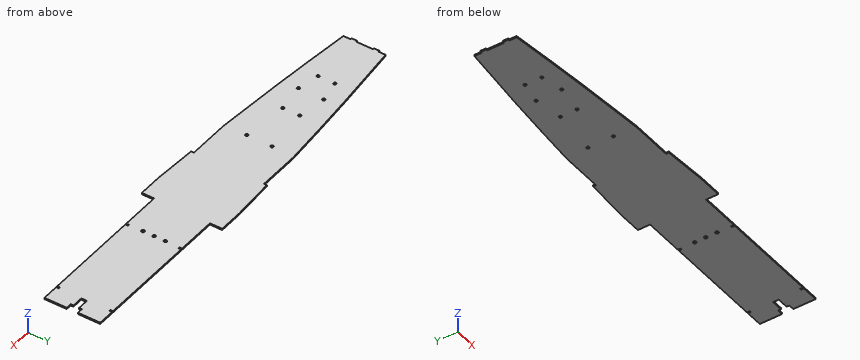
```python
from build123d import *

# Parameters (mm, degrees)
BOSS_EXTRUDE1_DEPTH    = 1.5875
CUT_EXTRUDE1_DEPTH     = 637.645771754
SKETCH4_W              = 1.5875
SKETCH4_H              = 3.175
CUT_EXTRUDE2_DEPTH     = 637.645771754
SKETCH6_W              = 47.338109293
SKETCH6_H              = 3.175
CUT_EXTRUDE3_DEPTH     = 637.645771754
SKETCH7_R              = 1.5875
ARTS4_MOUNT_DEPTH      = 637.645771754
SKETCH8_R              = 1.5875
TELEMETRUM_MOUNT_DEPTH = 637.645771754
SKETCH9_R              = 1.74625
CUT_EXTRUDE4_DEPTH     = 637.645771754


with BuildPart() as part:
    # Sketch1 → Boss-Extrude1 (new body)
    with BuildSketch(Plane.XY):
        with BuildLine():
            Line((508, -45.72), (508, -34.29))
            Line((508, -34.29), (635, -34.29))
            Line((635, -34.29), (635, 34.29))
            Line((635, 34.29), (508, 34.29))
            Line((508, 34.29), (508, 45.72))
            Line((508, 45.72), (429.947642932, 45.72))
            add(Edge.make_bspline(
                [(161.29, 23.981640211), (161.616784041, 24.018741883), (172.383373415, 25.239568053), (204.048179593, 28.679227521), (256.348102033, 33.727983978), (319.188209115, 38.915614913), (371.60802888, 42.52482202), (408.536828327, 44.644949518), (424.488578703, 45.455997775), (429.947642932, 45.72)],
                knots=[0.31962734, 0.31962734, 0.31962734, 0.31962734, 0.321557959, 0.383234508, 0.506587607, 0.629940705, 0.753293803, 0.814970352, 0.847054623, 0.847054623, 0.847054623, 0.847054623], degree=3))
            Line((161.29, 23.981640211), (161.29, 15.875))
            Line((161.29, 15.875), (159.7025, 15.875))
            Line((159.7025, 15.875), (159.7025, 9.525))
            Line((159.7025, 9.525), (161.29, 9.525))
            Line((161.29, 9.525), (161.29, -9.525))
            Line((161.29, -9.525), (159.7025, -9.525))
            Line((159.7025, -9.525), (159.7025, -15.875))
            Line((159.7025, -15.875), (161.29, -15.875))
            Line((161.29, -15.875), (161.29, -23.981640211))
            add(Edge.make_bspline(
                [(429.947642932, -45.72), (424.488578703, -45.455997775), (408.536828327, -44.644949518), (371.60802888, -42.52482202), (319.188209115, -38.915614913), (256.348102033, -33.727983978), (204.048179593, -28.679227521), (172.383373415, -25.239568053), (161.616784041, -24.018741883), (161.29, -23.981640211)],
                knots=[0.16612059, 0.16612059, 0.16612059, 0.16612059, 0.198204861, 0.25988141, 0.383234508, 0.506587607, 0.629940705, 0.691617254, 0.693547873, 0.693547873, 0.693547873, 0.693547873], degree=3))
            Line((429.947642932, -45.72), (508, -45.72))
        make_face()
    extrude(amount=BOSS_EXTRUDE1_DEPTH)

    # Sketch3 → Cut-Extrude1 (cut, through all)
    with BuildSketch(Plane.XY.offset(1.5875)):
        Polygon((635, 34.29), (508, 34.29), (508, 45.72), (457.2, 45.72), (457.2, 31.75), (635, 31.75), align=None)
        Polygon((508, -45.72), (508, -34.29), (635, -34.29), (635, -31.75), (457.2, -31.75), (457.2, -45.72), align=None)
        Polygon((628.65, 6.35), (628.65, 3.175), (615.95, 3.175), (615.95, -3.175), (628.65, -3.175), (628.65, -6.35), (635, -6.35), (635, 6.35), align=None)
    extrude(amount=-CUT_EXTRUDE1_DEPTH, mode=Mode.SUBTRACT)

    # Sketch4 → Cut-Extrude2 (cut, through all)
    with BuildSketch(Plane.XY.offset(1.5875)):
        with Locations((503.1105, 30.1625)):
            Rectangle(SKETCH4_W, SKETCH4_H)
        with Locations((615.15625, 30.1625)):
            Rectangle(SKETCH4_W, SKETCH4_H)
        with Locations((503.1105, -30.1625)):
            Rectangle(SKETCH4_W, SKETCH4_H)
        with Locations((615.15625, -30.1625)):
            Rectangle(SKETCH4_W, SKETCH4_H)
    extrude(amount=-CUT_EXTRUDE2_DEPTH, mode=Mode.SUBTRACT)

    # Sketch6 → Cut-Extrude3 (cut, through all)
    with BuildSketch(Plane.XY.offset(1.5875)):
        with Locations((357.330945353, 41.432202354)):
            Rectangle(SKETCH6_W, SKETCH6_H)
        with Locations((357.330945353, -41.432202354)):
            Rectangle(SKETCH6_W, SKETCH6_H)
    extrude(amount=-CUT_EXTRUDE3_DEPTH, mode=Mode.SUBTRACT)

    # Sketch7 → ARTS4 mount (cut, through all)
    with BuildSketch(Plane.XY.offset(1.5875)):
        with Locations((331.688780886, 14.478)):
            Circle(SKETCH7_R)
        with Locations((331.688780886, -14.478)):
            Circle(SKETCH7_R)
        with Locations((247.868780886, 14.478)):
            Circle(SKETCH7_R)
        with Locations((247.868780886, -14.478)):
            Circle(SKETCH7_R)
    extrude(amount=-ARTS4_MOUNT_DEPTH, mode=Mode.SUBTRACT)

    # Sketch8 → Telemetrum Mount (cut, through all)
    with BuildSketch(Plane.XY.offset(1.5875)):
        with Locations((280.018433255, 9.525)):
            Circle(SKETCH8_R)
        with Locations((280.018433255, -9.525)):
            Circle(SKETCH8_R)
        with Locations((222.893833255, -9.525)):
            Circle(SKETCH8_R)
        with Locations((222.893833255, 9.525)):
            Circle(SKETCH8_R)
    extrude(amount=-TELEMETRUM_MOUNT_DEPTH, mode=Mode.SUBTRACT)

    # Sketch9 → Cut-Extrude4 (cut, through all)
    with BuildSketch(Plane.XY.offset(1.5875)):
        with Locations((502.31675, -12.7)):
            Circle(SKETCH9_R)
        with Locations((502.31675, 12.7)):
            Circle(SKETCH9_R)
        with Locations((502.31675, 0)):
            Circle(SKETCH9_R)
    extrude(amount=-CUT_EXTRUDE4_DEPTH, mode=Mode.SUBTRACT)


solid = part.part
```
Can you work these out from the model? Positions are in its coordinate system, mm. Round coordinates to 2 decimals unless told otherwise and drop trailing zeros. Loops run counter-clockwise (first coordinate to the right, second up) from the corner with the lowest first, then second, coordinate; pieces in that order, holes last. Notation, with made-up numbers: M 88.5,5.5 L 123.5,5.5 A24 cw 123.5,37.5 Z; hole C -32.5,0 d11. An arc over 180 degrees is marked long. Write item = value, one per line. Start each with the question number.
(1) Suppose I cut it at B-B on x = 358.5. Write out the boundary of the cut face in (y, z), plus the area to 3 significant figures.
(2) Suppose I cut it at A-A on z = 0.4. Give the number of separate pieces and of enclosed holes in the cut face, plus the area to 3 significant figures.
(3) Suppose I cut it at C-C on x = 466. Write out the boundary of the cut face in (y, z), plus the area to 3 significant figures.
(4) I'm going to push flat-ended pins straight in: P1, Ø4, axis at x = 280.02, y = 9.52, coming from the +Z side; P2, Ø0.8, axis at y = -41, z = 1, coming from the +X side. Where does each tip first touch, or does it pass through?
(5) I need wall thicknesses on line 1 along Y through (x, z) = (224, 1.5); line 2 along X through (y, z) = (17, 0.65); line 3 along Y through (x, z) = (575, 0.1). Which ranges of each line are inside material? Lowest first, please.
Answer block:
q1.outline = M -39.84,0 L 39.84,0 L 39.84,1.59 L -39.84,1.59 Z
q1.area = 127 mm²
q2.separate_pieces = 1
q2.enclosed_holes = 11
q2.area = 32,900 mm²
q3.outline = M -31.75,0 L 31.75,0 L 31.75,1.59 L -31.75,1.59 Z
q3.area = 101 mm²
q4.P1 = 1.59
q4.P2 = 457.2
q5.line_1 = -30.57 to -10.66, -8.39 to 8.39, 10.66 to 30.57
q5.line_2 = 161.29 to 635
q5.line_3 = -31.75 to 31.75
